The figure shows three views and two pictorial views of one solid part (mm, origin at its lowest corner). Answer the questions. A direction names the side the tool comes from. Coordinates: 2 decimals unless noted, no trailing zeros. Order: outer loops, then holes, each group sorted by start corner. A loop starts at its lowest first (then second) coordinate and runs counter-clockwise, first axis right, second up. Notation, with made-up numbers: (-33.5, 12.25) -> (13.5, 12.25) arc R20 cw to (13.5, 27.25) -> close; hole circle Ø1 at (14.5, 81.25). An arc over 180 degrees is marked (long way). Use one line per item in the form item = value.
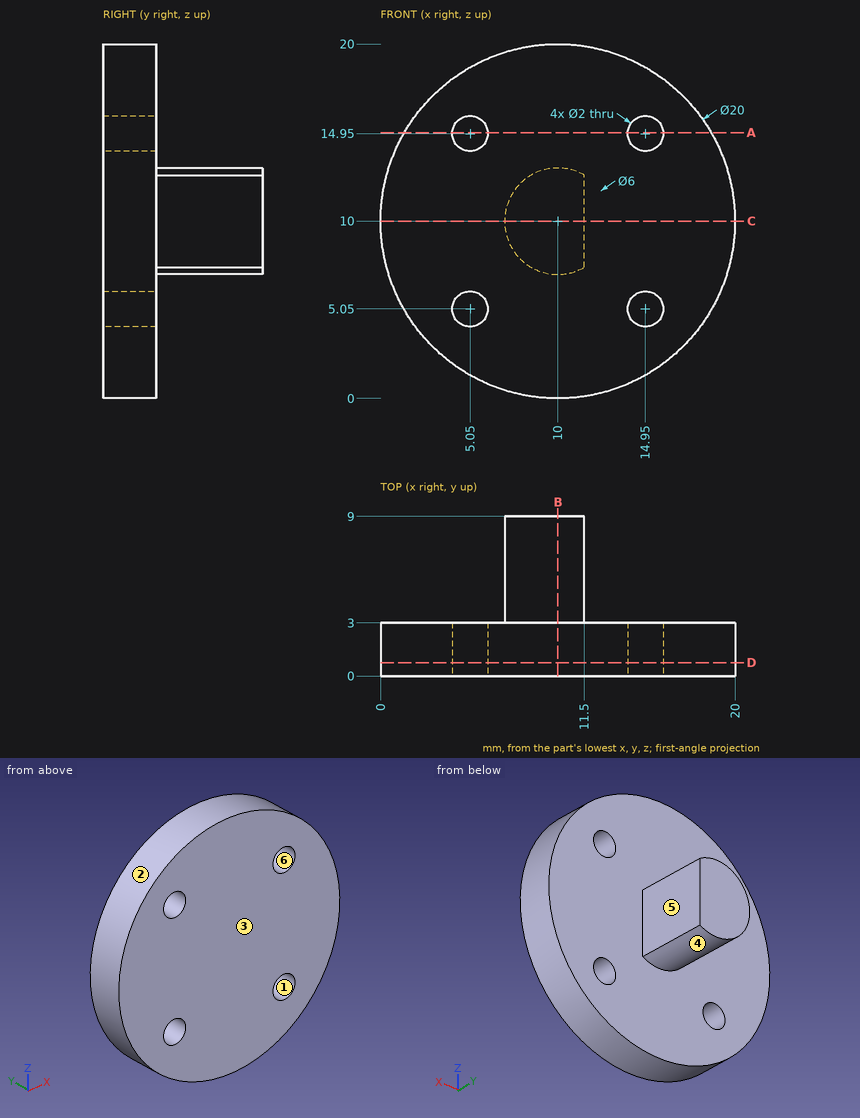
(1) The mould has two halves that part along X. Classify the marked faces 1, 2 and 3: released by +X, released by -X, zero draft, split by the parting line, or undercut.
Data:
face_1 = undercut
face_2 = split by the parting line
face_3 = zero draft
(2) Straight lines are drawn through the part: line 1 along Z through (x, y) = (14.25, 1.5) (1 decimal); line 2 along Z through (x, y) = (4.75, 0.5) (1 decimal); line 3 along Y through (x, z) = (14.5, 16.25). For each, find the intervals that lie inside material, in ascending order.
Data:
line_1 = 0.9 to 4.3, 5.8 to 14.2, 15.7 to 19.1
line_2 = 1.5 to 4.1, 6 to 14, 15.9 to 18.5
line_3 = 0 to 3
(3) Section D-D on y = 0.75 is taken. Write down the section's boundary in (x, z).
Data:
outline = circle Ø20 at (10, 10); hole circle Ø2 at (5.05, 5.05); hole circle Ø2 at (5.05, 14.95); hole circle Ø2 at (14.95, 5.05); hole circle Ø2 at (14.95, 14.95)
(4) Section A-A on z = 15 is taken. Write down the section's boundary in (x, y).
Data:
outline = (1.34, 0) -> (4.05, 0) -> (4.05, 3) -> (1.34, 3) -> close; (6.05, 0) -> (13.95, 0) -> (13.95, 3) -> (6.05, 3) -> close; (15.95, 0) -> (18.66, 0) -> (18.66, 3) -> (15.95, 3) -> close
(5) Which of the six approach directions +Z, -Z, +X, -X, +Y, -Y give full straight-line access (tool end or side, diameter ignored) to the marked faces 4, 5 and 6?
Data:
face_4 = +Y
face_5 = +Z, -Z, +X, +Y
face_6 = +Y, -Y
(6) Section C-C on z = 10 is taken. Write down the section's boundary in (x, y), plus the area to 3 significant figures.
Data:
outline = (0, 0) -> (20, 0) -> (20, 3) -> (11.5, 3) -> (11.5, 9) -> (7, 9) -> (7, 3) -> (0, 3) -> close
area = 87.0 mm²
(7) Section B-B on x = 10 is taken. Write down the section's boundary in (y, z), plus the area to 3 significant figures.
Data:
outline = (0, 0) -> (3, 0) -> (3, 7) -> (9, 7) -> (9, 13) -> (3, 13) -> (3, 20) -> (0, 20) -> close
area = 96.0 mm²
(8) Each of these flat-tipped pins is pushed along its axis until it touches: P1, Ø2.5, axis at x = 14.95, z = 14.95, coming from the +Y side; P2, Ø1.5, axis at y = 5, z = 6.5, coming from the +X side; P3, Ø1.5, axis at x = 4, y = 1.5, coming from the +Z side. Where does it stop, or does it pass through?
Data:
P1 = 3
P2 = 11.2
P3 = 18.51
